Geometry: final body of the model. Coordinates: model frame, mm. Face numbers are marked on the shaded views. A direction names the side the tool comes from. Give positions to 0.01 mm unless a question says otherwise; leave off trailing zeros. Loops run counter-clockwise (first coordinate to the right, second up) from the corner with the lowest first, then second, coordinate; pieces in that order, holes last.
```python
from build123d import *

# Parameters (mm, degrees)
EXTRUDE_1_DEPTH     = 15
EXTRUDE_2_DEPTH     = 15
SKETCH_3_R          = 1.75
CUT_EXTRUDE_1_DEPTH = 6


with BuildPart() as part:
    # Эскиз1 → Бобышка-Вытянуть1 (new body)
    with BuildSketch(Plane(origin=(0, 0, 0), x_dir=(1, 0, 0), z_dir=(0, 1, 0))):
        with BuildLine():
            Line((-5.773502692, 0), (-18.660254038, 0))
            Line((-18.660254038, 0), (-18.660254038, 5))
            Line((-18.660254038, 5), (-8.660254038, 5))
            ThreePointArc((-8.660254038, 5), (0, 10), (8.660254038, 5))
            Line((8.660254038, 5), (18.660254038, 5))
            Line((18.660254038, 5), (18.660254038, 0))
            Line((18.660254038, 0), (5.773502692, 0))
            Line((5.773502692, 0), (2.886751346, 5))
            Line((2.886751346, 5), (-2.886751346, 5))
            Line((-2.886751346, 5), (-5.773502692, 0))
        make_face()
    extrude(amount=EXTRUDE_1_DEPTH)

    # Эскиз2 → Бобышка-Вытянуть2 (add)
    with BuildSketch(Plane(origin=(0, 15, 0), x_dir=(1, 0, 0), z_dir=(0, 1, 0))):
        with BuildLine():
            Line((-18.660254038, 5), (-8.660254038, 5))
            ThreePointArc((-8.660254038, 5), (0, 10), (8.660254038, 5))
            Line((8.660254038, 5), (18.660254038, 5))
            Line((18.660254038, 5), (18.660254038, 0))
            Line((18.660254038, 0), (10, 0))
            Line((10, 0), (3, 0))
            ThreePointArc((3, 0), (0, 3), (-3, 0))
            Line((-3, 0), (-18.660254038, 0))
            Line((-18.660254038, 0), (-18.660254038, 5))
        make_face()
    extrude(amount=EXTRUDE_2_DEPTH)

    # Эскиз3 → Вырез-Вытянуть1 (cut, through all)
    with BuildSketch(Plane(origin=(0, 0, -5), x_dir=(-1, 0, 0), z_dir=(0, 0, -1))):
        with Locations((-13.660254038, 5)):
            Circle(SKETCH_3_R)
        with Locations((-13.660254038, 25)):
            Circle(SKETCH_3_R)
        with Locations((13.660254038, 5)):
            Circle(SKETCH_3_R)
        with Locations((13.660254038, 25)):
            Circle(SKETCH_3_R)
    extrude(amount=-CUT_EXTRUDE_1_DEPTH, mode=Mode.SUBTRACT)


solid = part.part
```
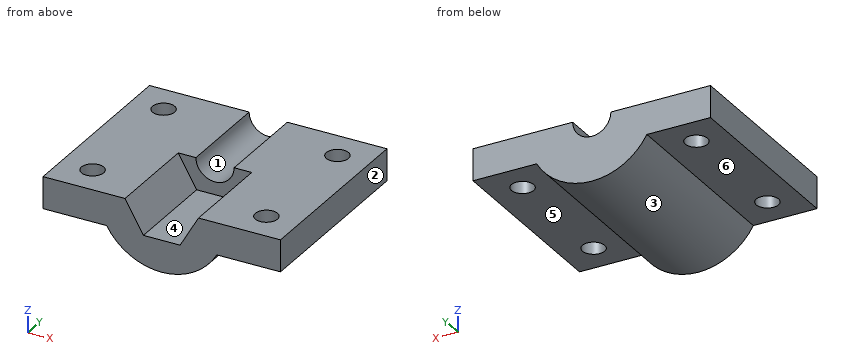
Q1. Pin query (flat end, axial travel): pin 1 Ø6.5 at (x, y) = (-0.5, 9) entering from +Z; pin 2 Ø3 at (x, y) = (-13, 16.5) entering from -Z; pin 3 Ø4 at (y, z) = (14.5, -8.5) entering from +X; pin 4 Ø5.5 at (x, y) = (-13.66, 25) entering from +Z. Return the tip coordinate at first contact, or that it passes through.
Q2. Reachability of the marked faces 4, 5 and 6 from +Z, -Z, +X, -X, +Y, -Y: full face, straight path, thin tool, end or side. Return the list, or none.
Q3. Section query C-C, the plane x = -13. Return loops of the section in (y, z).
Q4. Section query D-D, the plane y = 22.5. Return loops of the section in (x, z), and give its area (3 significant figures).
Q5. Section query B-B, the plane z = -2. Return loops of the section in (x, y).
Q6. Section query A-A, the plane y = 5. Return loops of the section in (x, z).
Q7. Mould query, pull axis X, two halves, no side actions, for the marked faces 1, 2 and 3. Classes: +X half, -X half, draft (parallel to the pull), parting line (faces both ways), or undercut.
Q8. Material intervals for probe 1 along Z at (x, y) = (-10, 22); probe 2 along X at (y, z) = (8.75, -3.75); probe 3 along Z at (x, y) = (-5, 19), sorted ascending.
Resolved:
1. pin 1: stops at z = -3.5
1. pin 2: stops at z = -5
1. pin 3: stops at x = 7.6
1. pin 4: stops at z = 0
2. face 4: +Z, -Y
2. face 5: -Z, +X, +Y, -Y
2. face 6: -Z, -X, +Y, -Y
3. outline: (0, -5) - (3.38, -5) - (3.38, 0) - (0, 0) - close; (6.62, -5) - (23.38, -5) - (23.38, 0) - (6.62, 0) - close; (26.62, -5) - (30, -5) - (30, 0) - (26.62, 0) - close
4. outline: (-18.66, -5) - (-8.66, -5) arc R10 ccw to (8.66, -5) - (18.66, -5) - (18.66, 0) - (3, 0) arc R3 cw to (-3, 0) - (-18.66, 0) - close
4. area: 234 mm2
5. outline: (-18.66, 0) - (-4.62, 0) - (-4.62, 15) - (-2.24, 15) - (-2.24, 30) - (-18.66, 30) - close; (2.24, 15) - (4.62, 15) - (4.62, 0) - (18.66, 0) - (18.66, 30) - (2.24, 30) - close; hole circle Ø3.5 at (-13.66, 5); hole circle Ø3.5 at (-13.66, 25); hole circle Ø3.5 at (13.66, 5); hole circle Ø3.5 at (13.66, 25)
6. outline: (-18.66, -5) - (-15.41, -5) - (-15.41, 0) - (-18.66, 0) - close; (-11.91, -5) - (-8.66, -5) arc R10 ccw to (8.66, -5) - (11.91, -5) - (11.91, 0) - (5.77, 0) - (2.89, -5) - (-2.89, -5) - (-5.77, 0) - (-11.91, 0) - close; (15.41, -5) - (18.66, -5) - (18.66, 0) - (15.41, 0) - close
7. face 1: undercut
7. face 2: +X half
7. face 3: parting line
8. probe 1: z = -5 to 0
8. probe 2: x = -18.66 to -3.61, 3.61 to 18.66
8. probe 3: z = -8.66 to 0
